Model file for the job. Use its own axes, mm. A direction names the side the tool comes from. Coordinates: 2 decimals unless noted, no trailing zeros. Order: outer loops, then holes, each group sorted by start corner. A loop starts at its lowest first (then second) coordinate and runs counter-clockwise, first axis right, second up. Notation, with made-up numbers: M 6.25,-20.75 L 65.25,-20.75 A7 ccw 65.25,-8.75 Z; hole C 29,9 d2. An arc over 180 degrees is marked long. Return JSON: item names as keys, results as strings.
Autodesk Inventor part; units mm, degrees
ref_plane "YZ Plane" through (0, 0, 0) normal (1, 0, 0) x (0, 1, 0)
ref_plane "XZ Plane" through (0, 0, 0) normal (0, 1, 0) x (-1, 0, 0)
ref_plane "XY Plane" through (0, 0, 0) normal (0, 0, 1) x (1, 0, 0)
sketch "Boceto1" plane through (0, 0, 0) normal (0, 0, 1) x (1, 0, 0)
  line L0 (13, 15.1987) -> (13, -15.1987)
  arc A0 (13, 15.1987) -> (-13, 15.1987) centre (0, 0) ccw
  line L1 (-10.89, 14.1053) -> (-10.89, -14.1053)
  arc A1 (10.89, 14.1053) -> (-10.89, 14.1053) centre (0, 0) ccw
  line L2 (-13, -15.1987) -> (-13, 15.1987)
  arc A2 (-10.89, -14.1053) -> (10.89, -14.1053) centre (0, 0) ccw
  arc A3 (-13, -15.1987) -> (13, -15.1987) centre (0, 0) ccw
  line L3 (10.89, 14.1053) -> (10.89, -14.1053)
  line L4 (-9.6976, 12.5455) -> (-9.6976, -12.3312)
  arc A4 (9.5084, 12.5455) -> (-9.6976, 12.5455) centre (-0.0946, 0.1071) ccw
  arc A5 (-9.6976, -12.3312) -> (9.5084, -12.3312) centre (-0.0946, 0.1071) ccw
  line L5 (9.5084, 12.5455) -> (9.5084, -12.3312)
extrude "Extrusión1" add sketch "Boceto1" along normal blind 5 contours A1 L3 A2 L1
sketch "Boceto2" plane through (0, 0, 0) normal (0, 0, -1) x (-1, 0, 0)
  arc A0 (-9.5084, -12.3312) -> (9.6976, -12.3312) centre (0.0946, 0.1071) ccw
  arc A1 (-10.89, -14.1053) -> (10.89, -14.1053) centre (0, 0) ccw
  arc A2 (13.13, 15.0742) -> (-12.87, 15.0742) centre (0.13, -0.1245) ccw
  arc A3 (-12.87, -15.0742) -> (12.87, -15.0742) centre (0, 0.2347) ccw
  circle A4 centre (0, 0) radius 20
  line L0 (-12.87, -15.0742) -> (-12.87, -12.3254)
  line L1 (-12.87, 12.3254) -> (-12.87, 15.0742)
  line L2 (12.87, 12.3254) -> (13, 9.0726)
  line L3 (12.87, -12.3254) -> (12.87, -15.0742)
  dimension "d2" = 40
extrude "Extrusión2" add sketch "Boceto2" along normal blind 3
sketch "Boceto3" plane through (0, 0, -3) normal (0, 0, -1) x (-1, 0, 0)
  arc A0 (0.9994, -13.463) -> (-0.9994, -13.463) centre (0, 0) ccw
  arc A1 (-0.9994, -13.463) -> (0.9994, -13.463) centre (0, -13.4987) ccw
  dimension "d5" = 27
  dimension "d6" = 2
extrude "Extrusión3" cut sketch "Boceto3" against normal blind 0.5
hole "Hole1" at (-0.23, -7.8199, -2.5) direction (0, 0, 1) diameter 2 end through all
equation "\"d16\" = Grosor"
equation "\"Radio_pliegue\" = Grosor"
equation "\"Anchura_desahogo_plegado\" = Grosor"
equation "\"Profundidad_desahogo_plegado\" = 0.5 * Grosor"
equation "\"Tamaño_destalonado\" = 4 * Grosor"
equation "\"Remanente_mínimo\" = 2 * Grosor"
equation "\"Radiodetransición\" = Radio_pliegue"
equation "\"Tamaño_de_radio_de_Jacobi\" = Radio_pliegue"
equation "\"TamañoSeparación\" = Grosor"
properties part number "Tapa 3"
Item 1: Saw through at D-D (y = -8). Write the cut outline in (x, z), and give its area (3 significant figures).
Check result:
{"outline": "M -18.33,-3 L -10.87,-3 L -10.87,-2.5 L -1.21,-2.5 L -1.21,0 L -9.7,0 L -9.7,5 L -10.89,5 L -10.89,0 L -18.33,0 Z; M 0.75,-2.5 L 10.87,-2.5 L 10.87,-3 L 18.33,-3 L 18.33,0 L 10.89,0 L 10.89,5 L 9.51,5 L 9.51,0 L 0.75,0 Z", "area": "107 mm2"}
Item 2: Saw through at A-A (z = 2.75). Write the cut outline in (x, y), and give its area (3 significant figures).
Check result:
{"outline": "M -10.89,-14.11 A17.82 ccw 10.89,-14.11 L 10.89,14.11 A17.82 ccw -10.89,14.11 Z; hole M -9.7,-12.33 A15.71 ccw 9.51,-12.33 L 9.51,12.55 A15.71 ccw -9.7,12.55 Z", "area": "161 mm2"}
Item 3: Pull direction Y, two halves, no side cores. Call faces 1 (the flat face through (10, 0, 5)), 2 (the cylindrical face through (0.16, -17.82, 2.46)), 3 (the flat face through (-9.698, 0, 2)), 4 (the cylindrical face through (-0.58, 13.488, -2.754)): +Y half, -Y half, draft (parallel to the pull), parting line (faces both ways), or undercut.
Check result:
{"face 1": "draft", "face 2": "-Y half", "face 3": "undercut", "face 4": "undercut"}
Item 4: Drop flat-ended pins along their axis: pin 1 Ø2 at (x, y) = (-4.5, 14) entering from +Z; pin 2 Ø8 at (x, y) = (4, -7) entering from -Z; pin 3 Ø2.5 at (y, z) = (3.5, 1.5) entering from -X. Give the stop position or say it passes through.
Check result:
{"pin 1": "stops at z = 0", "pin 2": "stops at z = -2.5", "pin 3": "stops at x = -10.89"}
Item 5: 3-axis set-ups, long thin cutter, end or side, ignore diameter. For faces 5 (the cylindrical face through (-0.16, 17.82, 2.46)), 6 (the flat face through (9.508, 0, 2)), 7 (the flat face through (0, 0, -2.5)), 8 (the flat face through (10.89, 0, 2)): which of +Z, -Z, +X, -X, +Y, -Y reach the whole face in a straight line?
Check result:
{"face 5": "+Z, +Y", "face 6": "+Z", "face 7": "-Z", "face 8": "+Z, +X, +Y, -Y"}
Item 6: Saw through at C-C (x = -0.23). Write the cut outline in (y, z).
Check result:
{"outline": "M -20,-3 L -14.47,-3 L -14.47,-2.5 L -8.82,-2.5 L -8.82,0 L -15.61,0 L -15.61,5 L -17.82,5 L -17.82,0 L -20,0 Z; M -6.82,-2.5 L 13.5,-2.5 L 13.5,-3 L 20,-3 L 20,0 L 17.82,0 L 17.82,5 L 15.82,5 L 15.82,0 L -6.82,0 Z"}
Item 7: Wall check: line 1 (X direction, y = 7.5, z = 1.5); line 2 (Y direction, x = 0, z = -2.65); line 3 (Y direction, x = -0.5, z = 1.5). Give the ranges that are in metal, low to high.
Check result:
{"line 1": "x = -10.89 to -9.7, 9.51 to 10.89", "line 2": "y = -20 to -14.5, 13.5 to 20", "line 3": "y = -17.81 to -15.6, 15.82 to 17.81"}
Item 8: Saw through at B-B (y = 0). Write the cut outline in (x, z), and give its area (3 significant figures).
Check result:
{"outline": "M -20,-3 L -13.5,-3 L -13.5,-2.5 L 13.5,-2.5 L 13.5,-3 L 20,-3 L 20,0 L 10.89,0 L 10.89,5 L 9.51,5 L 9.51,0 L -9.7,0 L -9.7,5 L -10.89,5 L -10.89,0 L -20,0 Z", "area": "119 mm2"}
